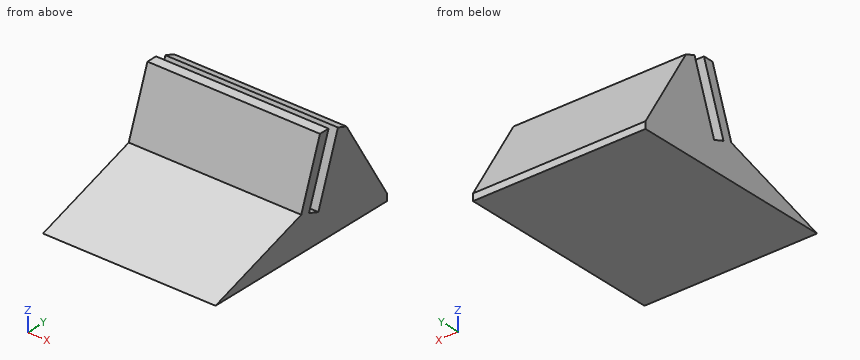
```python
from build123d import *

# Parameters (mm, degrees)
ESQUISSE1_W        = 50
ESQUISSE1_H        = 30
BOSS_EXTRU_1_DEPTH = 2
BOSS_EXTRU_2_DEPTH = 50
BOSS_EXTRU_4_DEPTH = 50


with BuildPart() as part:
    # Esquisse1 → Boss.-Extru.1 (new body)
    with BuildSketch(Plane.XY):
        with Locations((25, 15)):
            Rectangle(ESQUISSE1_W, ESQUISSE1_H)
    extrude(amount=BOSS_EXTRU_1_DEPTH)

    # Esquisse2 → Boss.-Extru.2 (add)
    with BuildSketch(Plane(origin=(50, 0, 0), x_dir=(0, 0, -1), z_dir=(1, 0, 0))):
        Polygon((-2, 0), (-10, 0), (-27.990922917, 6.548160429), (-27.990922917, 9.548160429), (-9.197070502, 2.707757562), (-8, 5.996681735), (-26.793852416, 12.837084602), (-25.701941713, 15.837084602), (-2, 30), align=None)
    extrude(amount=-BOSS_EXTRU_2_DEPTH)

    # Esquisse4 → Boss.-Extru.4 (add)
    with BuildSketch(Plane(origin=(50, 0, 0), x_dir=(0, 0, -1), z_dir=(1, 0, 0))):
        Polygon((0, 0), (0, -30), (-10, 0), align=None)
    extrude(amount=-BOSS_EXTRU_4_DEPTH)


solid = part.part
```
Work out the finished part from the listing and answer in its coordinate system (mm). Round coordinates to 2 decimals unless told otherwise and drop trailing zeros. Order: outer loops, then holes, each group sorted by start corner. A loop starts at its lowest first (then second) coordinate and runs counter-clockwise, first axis right, second up.
Q1. A cutting plane is placed at A-A, the plane z = 11.5. Determine the outline of the cut face in (x, y).
Solution:
outline: (0, 0.55) - (50, 0.55) - (50, 3.55) - (0, 3.55) - close; (0, 7.27) - (50, 7.27) - (50, 24.32) - (0, 24.32) - close
Q2. Find the intervals of material crossed by line 1 along Y through (x, z) = (41, 19.75); line 2 along Y through (x, z) = (22, 15); line 3 along Z through (x, y) = (41.5, -8), in increasing order.
Solution:
line 1: y = 3.55 to 6.55, 10.27 to 19.39
line 2: y = 1.82 to 4.82, 8.54 to 22.23
line 3: z = 0 to 7.33
Q3. A cutting plane is placed at D-D, the plane y = -3. Determine the outline of the cut face in (x, z), then the cut area to 3 significant figures.
Solution:
outline: (0, 0) - (50, 0) - (50, 9) - (0, 9) - close
area: 450 mm2
Q4. A cutting plane is placed at C-C, the plane z = 24.25. Determine the outline of the cut face in (x, y), then the cut area to 3 significant figures.
Solution:
outline: (0, 5.19) - (50, 5.19) - (50, 8.19) - (0, 8.19) - close; (0, 11.91) - (50, 11.91) - (50, 16.7) - (0, 16.7) - close
area: 390 mm2
Q5. Given pin 1 Ø1 at (x, z) = (33.5, 9.5) entering from +Y; pin 2 Ø1.5 at (x, y) = (22, -21) entering from +Z; pin 3 Ø5 at (x, z) = (40.5, 20) entering from +Y; pin 4 Ø6 at (y, z) = (9, 23.5) entering from +X, each flat-ended and moving along its own axis, determine where each tip first touches the part or whether it passes through.
Solution:
pin 1: stops at y = 25.82
pin 2: stops at z = 3.25
pin 3: stops at y = 20.74
pin 4: stops at x = 50
Q6. A cutting plane is placed at B-B, the plane x = 20. Determine the outline of the cut face in (y, z), then the cut area to 3 significant figures.
Solution:
outline: (-30, 0) - (30, 0) - (30, 2) - (15.84, 25.7) - (12.84, 26.79) - (6, 8) - (2.71, 9.2) - (9.55, 27.99) - (6.55, 27.99) - (0, 10) - close
area: 653 mm2
